Source: CAD feature listing. Evaluate the final solid. Frame: model axes, mm. Face numbers are marked on the shaded views. A direction names the side the tool comes from. Coordinates: 2 decimals unless noted, no trailing zeros. Loops run counter-clockwise (first coordinate to the right, second up) from the corner with the lowest first, then second, coordinate; pieces in that order, holes last.
from build123d import *


with BuildPart() as part:
    # 草图1 → 旋转1 (revolve)
    with BuildSketch(Plane.XY):
        Polygon((-10.764397906, 0), (37.235602094, 0), (37.235602094, 3.5), (36.735602094, 4), (33.235602094, 4), (33.235602094, 3.8), (32.235602094, 3.8), (32.235602094, 3.95), (32.235602094, 5), (28.235602094, 5), (28.235602094, 6), (19.835602094, 6), (19.835602094, 5.5), (18.735602094, 5.5), (18.735602094, 6), (3.235602094, 6), (3.235602094, 7), (1.235602094, 7), (1.235602094, 6), (-1.764397906, 6), (-1.764397906, 5), (-5.764397906, 5), (-5.764397906, 3.95), (-5.764397906, 3.8), (-6.764397906, 3.8), (-6.764397906, 4), (-10.264397906, 4), (-10.764397906, 3.5), align=None)
    revolve(axis=Axis((-10.764397906, 0, 0), (1, 0, 0)))


solid = part.part
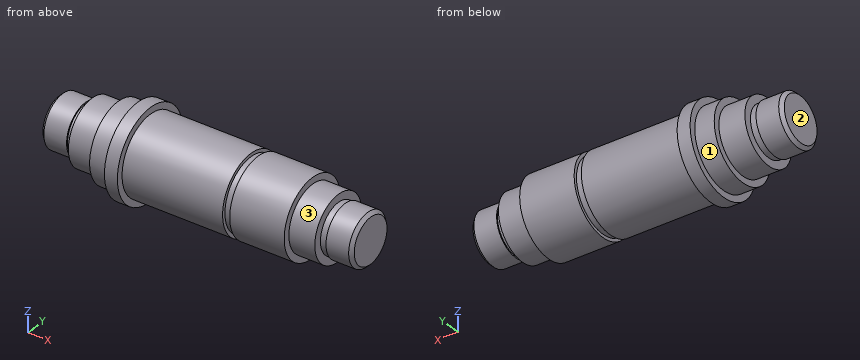
Q1. Access query for the marked faces 1, 2 and 3. Directions: +Z, -Z, +X, -X, +Y, -Y. A direction counts if a zero-diameter tool reaches every point of the face in a straight line with its end or side. Return the directions, or none.
Q2. Section A-A, the plane x = 21.5. Return the cut outline in (y, z), plus the area to 3 significant figures.
Q3. Line query: line 1 along X through (y, z) = (2.75, -3); line 2 along Z through (x, y) = (35, 1.25); line 3 along X through (y, z) = (-5.25, 3). Output: solid intervals per line, ascending.
Q4. Contact query for flat-ended pins moving along their axis: pin 1 Ø3 at (x, z) = (22, 4.5) entering from -Y; pin 2 Ø3 at (x, y) = (-3.5, -3) entering from +Z; pin 3 Ø5 at (x, y) = (8, -4.5) entering from +Z; pin 4 Ø6 at (y, z) = (1, 4.5) entering from -X. Output: stop coordinate, or through.
Derived:
1. face 1: -X
1. face 2: +Z, -Z, -X, +Y, -Y
1. face 3: +X
2. outline: circle Ø12 at (0, 0)
2. area: 113 mm2
3. line 1: x = -5.76 to 32.24
3. line 2: z = -3.8 to 3.8
3. line 3: x = 1.24 to 3.24
4. pin 1: stops at y = -5.2
4. pin 2: stops at z = 4.77
4. pin 3: stops at z = 5.66
4. pin 4: stops at x = -10.76
